Geometry check sheet. Reference: the model listing, model coordinates, mm. Coordinates: 2 decimals unless noted, no trailing zeros. Loops run counter-clockwise (first coordinate to the right, second up) from the corner with the lowest first, then second, coordinate; pieces in that order, holes last.
from build123d import *

# Parameters (mm, degrees)
F1_DEPTH  = 5.08
F2_DEPTH  = 5.08
F3_W      = 124.8834840953
F3_H      = 134.0803280473
F4_DEPTH  = 25.4
F5_DEPTH  = 1.27
F6_DEPTH  = 1.27
F8_DEPTH  = 25.4
F9_DEPTH  = 2.54
F10_DEPTH = 2.54
F11_SIZE2 = 3.418656578
F11_SIZE  = 5.6896
F12_SIZE2 = 3.6576
F12_SIZE  = 5.6322100916


with BuildPart() as f1:
    # F0 (on Front) → F1 (new body)
    with BuildSketch(Plane.XZ):
        with BuildLine():
            add(Edge.make_bspline(
                [(11.6870266183, 8.3659507286), (11.9476031572, 8.1243832132), (12.5616108346, 7.4348870399), (13.3502602627, 5.9055860485), (12.8304196463, 2.6136928469), (12.1032885822, -3.9726756525), (11.7671016032, -8.6546761386), (11.3077259518, -11.7183290107), (11.0820746049, -13.2232354954)],
                knots=[0.7644347581, 0.7644347581, 0.7644347581, 0.7644347581, 0.7813803339, 0.8102561854, 0.8494051355, 0.9057589485, 0.9537075591, 1, 1, 1, 1], degree=3))
            Line((11.6870266183, 8.3659507286), (10.7098612934, -7.1798651479))
            Line((10.7098612934, -7.1798651479), (-10.6029463932, 18.994666636))
            Line((-10.6029463932, 18.994666636), (-7.8187826003, 81.9431145827))
            add(Edge.make_bspline(
                [(-10.6029463932, 84.9773436785), (-9.8645957866, 84.411917966), (-8.8470388386, 83.6326772405), (-8.0272766718, 82.3316307612), (-7.8187826003, 81.9431145827)],
                knots=[0, 0, 0, 0, 0.0369842854, 0.0509698458, 0.0509698458, 0.0509698458, 0.0509698458], degree=3))
            add(Edge.make_bspline(
                [(-11.1952358857, -13.2855195552), (-11.1963398761, -12.8902117283), (-11.1997561984, -11.6669231231), (-11.1512885463, -5.3731858959), (-11.3422819981, 1.4393792063), (-12.1461643066, 4.6189611976), (-13.2850553088, 9.1238655935), (-15.2318124981, 13.6348809881), (-16.5294824008, 17.2010053959), (-19.3261405399, 23.6368379744), (-19.7379489625, 26.452730971), (-18.8574929103, 31.5305578619), (-16.6797816611, 35.2468825016), (-14.5909185063, 40.6408371255), (-13.4119591393, 46.1621954132), (-12.5394588361, 53.3896491248), (-12.0546254183, 59.9791874234), (-12.4642284532, 65.9827168693), (-12.3457592591, 73.9226808987), (-11.3164428193, 80.5227149139), (-11.5649092387, 84.7450814286), (-10.8268692537, 84.9232783602), (-10.6029463932, 84.9773436785)],
                knots=[0, 0, 0, 0, 0.0273896804, 0.0847579572, 0.1451631407, 0.1862204743, 0.2349457062, 0.2850522094, 0.3309978555, 0.390291, 0.4296935499, 0.4796750401, 0.527816225, 0.5818528524, 0.6365092781, 0.6980539867, 0.7565756752, 0.8124783975, 0.8767822708, 0.9378286387, 0.9811370802, 1, 1, 1, 1], degree=3))
            Line((-11.1952358857, -13.2855195552), (10.8409429303, -13.2855195552))
            add(Edge.make_bspline(
                [(10.8409429303, -13.2855195552), (10.9216527758, -13.2575733481), (11.0020770139, -13.2366740148), (11.0820746049, -13.2232354954)],
                knots=[0.9988692567, 0.9988692567, 0.9988692567, 0.9988692567, 1, 1, 1, 1], degree=3))
        make_face()
        with BuildLine():
            Line((10.7098612934, -7.1798651479), (11.6870266183, 8.3659507286))
            add(Edge.make_bspline(
                [(-7.8187826003, 81.9431145827), (-7.3326835412, 81.037298185), (-6.246332701, 78.0877738667), (-5.7619281696, 71.7972152113), (-5.7903461619, 61.0472196354), (-5.6098025476, 47.5528084715), (-5.6232359348, 35.7951775922), (-6.6035814728, 31.5572406566), (-6.642373723, 26.8588973108), (-4.7217209893, 21.7576733197), (-2.3324429206, 17.8568763905), (-0.0644904347, 14.9988475653), (2.1698029367, 12.9502128359), (5.7523840475, 11.2499433455), (8.6363164493, 10.2542124123), (10.6765655712, 9.2073747067), (11.4911211984, 8.5475648745), (11.6870266183, 8.3659507286)],
                knots=[0.0509698458, 0.0509698458, 0.0509698458, 0.0509698458, 0.0835768534, 0.1402547932, 0.2115954168, 0.293701069, 0.3674969806, 0.4121442254, 0.4580916534, 0.50894046, 0.5557476766, 0.5967458601, 0.6345135251, 0.6775157549, 0.7161326985, 0.7516948155, 0.7644347581, 0.7644347581, 0.7644347581, 0.7644347581], degree=3))
            Line((-7.8187826003, 81.9431145827), (-10.6029463932, 18.994666636))
            Line((-10.6029463932, 18.994666636), (10.7098612934, -7.1798651479))
        make_face()
        with BuildLine():
            Line((11.0820746049, -15.9663576633), (11.0820746049, -13.2855195552))
            Line((11.0820746049, -13.2855195552), (10.8409429303, -13.2855195552))
            add(Edge.make_bspline(
                [(8.3953980002, -15.9663576633), (9.1364610409, -14.6227373643), (10.004055933, -13.5752960653), (10.8409429303, -13.2855195552)],
                knots=[0.9871444865, 0.9871444865, 0.9871444865, 0.9871444865, 0.9988692567, 0.9988692567, 0.9988692567, 0.9988692567], degree=3))
            Line((8.3953980003, -15.9663576633), (11.0820746049, -15.9663576633))
        make_face()
        with BuildLine():
            add(Edge.make_bspline(
                [(8.3953980002, -15.9663576633), (9.1364610409, -14.6227373643), (10.004055933, -13.5752960653), (10.8409429303, -13.2855195552)],
                knots=[0.9871444865, 0.9871444865, 0.9871444865, 0.9871444865, 0.9988692567, 0.9988692567, 0.9988692567, 0.9988692567], degree=3))
            Line((10.8409429303, -13.2855195552), (-11.1952358857, -13.2855195552))
            Line((-11.1952358857, -13.2855195552), (-11.0308257863, -15.9663576633))
            Line((-11.0308257863, -15.9663576633), (8.3953980003, -15.9663576633))
        make_face()
        with BuildLine():
            Line((11.0820746049, -13.2855195552), (11.0820746049, -13.2232354954))
            add(Edge.make_bspline(
                [(10.8409429303, -13.2855195552), (10.9216527758, -13.2575733481), (11.0020770139, -13.2366740148), (11.0820746049, -13.2232354954)],
                knots=[0.9988692567, 0.9988692567, 0.9988692567, 0.9988692567, 1, 1, 1, 1], degree=3))
            Line((10.8409429303, -13.2855195552), (11.0820746049, -13.2855195552))
        make_face()
    extrude(amount=F1_DEPTH)

    # F2 (add): a face of the model
    f2_faces = [f1.faces().sort_by_distance(p)[0] for p in [
        (-5.0809274024, 0, 19.1888153538),
    ]]
    extrude(f2_faces, amount=F2_DEPTH)

    # F3 (on face) → F4 (cut)
    with BuildSketch(Plane.XZ.offset(5.08)):
        with Locations((7.2313416749, 30.1963053644)):
            Rectangle(F3_W, F3_H)
        with BuildLine():
            Line((-11.0308257863, -15.9663576633), (-11.1952358857, -13.2855195552))
            add(Edge.make_bspline(
                [(-11.1952358857, -13.2855195552), (-11.1963398761, -12.8902117283), (-11.1997561984, -11.6669231231), (-11.1512885463, -5.3731858959), (-11.3422819981, 1.4393792063), (-12.1461643066, 4.6189611976), (-13.2850553088, 9.1238655935), (-15.2318124981, 13.6348809881), (-16.5294824008, 17.2010053959), (-19.3261405399, 23.6368379744), (-19.7379489625, 26.452730971), (-18.8574929103, 31.5305578619), (-16.6797816611, 35.2468825016), (-14.5909185063, 40.6408371255), (-13.4119591393, 46.1621954132), (-12.5394588361, 53.3896491248), (-12.0546254183, 59.9791874234), (-12.4642284532, 65.9827168693), (-12.3457592591, 73.9226808987), (-11.3164428193, 80.5227149139), (-11.5649092387, 84.7450814286), (-10.8268692537, 84.9232783602), (-10.6029463932, 84.9773436785)],
                knots=[0, 0, 0, 0, 0.0273896804, 0.0847579572, 0.1451631407, 0.1862204743, 0.2349457062, 0.2850522094, 0.3309978555, 0.390291, 0.4296935499, 0.4796750401, 0.527816225, 0.5818528524, 0.6365092781, 0.6980539867, 0.7565756752, 0.8124783975, 0.8767822708, 0.9378286387, 0.9811370802, 1, 1, 1, 1], degree=3))
            add(Edge.make_bspline(
                [(11.0820746049, -13.2232354954), (11.3077259518, -11.7183290107), (11.7671016032, -8.6546761386), (12.1032885822, -3.9726756525), (12.8304196463, 2.6136928469), (13.3502602627, 5.9055860485), (12.443365527, 7.6641811468), (11.0743289472, 9.0032850711), (8.6363164493, 10.2542124123), (5.7523840475, 11.2499433455), (2.1698029367, 12.9502128359), (-0.0644904347, 14.9988475653), (-2.3324429206, 17.8568763905), (-4.7217209893, 21.7576733197), (-6.642373723, 26.8588973108), (-6.6035814728, 31.5572406566), (-5.6232359348, 35.7951775922), (-5.6098025476, 47.5528084715), (-5.7903461619, 61.0472196354), (-5.7619281696, 71.7972152113), (-6.2885094778, 78.6354885776), (-8.1960757736, 83.1341725308), (-9.8645957866, 84.411917966), (-10.6029463932, 84.9773436785)],
                knots=[0.7644347581, 0.7644347581, 0.7644347581, 0.7644347581, 0.810727199, 0.8586758096, 0.9150296226, 0.9541785727, 0.9830544242, 1.0127399426, 1.0483020596, 1.0869190032, 1.1299212329, 1.167688898, 1.2086870814, 1.2554942981, 1.3063431047, 1.3522905327, 1.3969377775, 1.470733689, 1.5528393413, 1.6241799649, 1.6808579047, 1.7274504726, 1.7644347581, 1.7644347581, 1.7644347581, 1.7644347581], degree=3))
            Line((11.0820746049, -13.2232354954), (11.0820746049, -15.9663576633))
            Line((11.0820746049, -15.9663576633), (-11.0308257863, -15.9663576633))
        make_face(mode=Mode.SUBTRACT)
        with BuildLine():
            add(Edge.make_bspline(
                [(-11.1952358857, -13.2855195552), (-11.1963398761, -12.8902117283), (-11.1997561984, -11.6669231231), (-11.1512885463, -5.3731858959), (-11.3422819981, 1.4393792063), (-12.1461643066, 4.6189611976), (-13.2850553088, 9.1238655935), (-15.2318124981, 13.6348809881), (-16.5294824008, 17.2010053959), (-19.3261405399, 23.6368379744), (-19.7379489625, 26.452730971), (-18.8574929103, 31.5305578619), (-16.6797816611, 35.2468825016), (-14.5909185063, 40.6408371255), (-13.4119591393, 46.1621954132), (-12.5394588361, 53.3896491248), (-12.0546254183, 59.9791874234), (-12.4642284532, 65.9827168693), (-12.3457592591, 73.9226808987), (-11.3164428193, 80.5227149139), (-11.5649092387, 84.7450814286), (-10.8268692537, 84.9232783602), (-10.6029463932, 84.9773436785)],
                knots=[0, 0, 0, 0, 0.0273896804, 0.0847579572, 0.1451631407, 0.1862204743, 0.2349457062, 0.2850522094, 0.3309978555, 0.390291, 0.4296935499, 0.4796750401, 0.527816225, 0.5818528524, 0.6365092781, 0.6980539867, 0.7565756752, 0.8124783975, 0.8767822708, 0.9378286387, 0.9811370802, 1, 1, 1, 1], degree=3))
            Line((-11.1952358857, -13.2855195552), (-11.0308257863, -15.9663576633))
            Line((-11.0308257863, -15.9663576633), (11.0820746049, -15.9663576633))
            Line((11.0820746049, -15.9663576633), (11.0820746049, -13.2232354954))
            add(Edge.make_bspline(
                [(11.0820746049, -13.2232354954), (11.3077259518, -11.7183290107), (11.7671016032, -8.6546761386), (12.1032885822, -3.9726756525), (12.8304196463, 2.6136928469), (13.3502602627, 5.9055860485), (12.443365527, 7.6641811468), (11.0743289472, 9.0032850711), (8.6363164493, 10.2542124123), (5.7523840475, 11.2499433455), (2.1698029367, 12.9502128359), (-0.0644904347, 14.9988475653), (-2.3324429206, 17.8568763905), (-4.7217209893, 21.7576733197), (-6.642373723, 26.8588973108), (-6.6035814728, 31.5572406566), (-5.6232359348, 35.7951775922), (-5.6098025476, 47.5528084715), (-5.7903461619, 61.0472196354), (-5.7619281696, 71.7972152113), (-6.2885094778, 78.6354885776), (-8.1960757736, 83.1341725308), (-9.8645957866, 84.411917966), (-10.6029463932, 84.9773436785)],
                knots=[0.7644347581, 0.7644347581, 0.7644347581, 0.7644347581, 0.810727199, 0.8586758096, 0.9150296226, 0.9541785727, 0.9830544242, 1.0127399426, 1.0483020596, 1.0869190032, 1.1299212329, 1.167688898, 1.2086870814, 1.2554942981, 1.3063431047, 1.3522905327, 1.3969377775, 1.470733689, 1.5528393413, 1.6241799649, 1.6808579047, 1.7274504726, 1.7644347581, 1.7644347581, 1.7644347581, 1.7644347581], degree=3))
        make_face()
        Polygon((-7.6687936671, 0), (0, 12.9914516583), (7.6687936671, 0), (0, -13.0022913218), align=None, mode=Mode.SUBTRACT)
    extrude(amount=-F4_DEPTH, mode=Mode.SUBTRACT)

    # F5 (add): a face of the model
    f5_faces = [f1.faces().sort_by_distance(p)[0] for p in [
        (0, -5.08, -0.0036132211),
    ]]
    extrude(f5_faces, amount=F5_DEPTH)

    # F6 (add): a face of the model
    f6_faces = [f1.faces().sort_by_distance(p)[0] for p in [
        (0, 5.08, -0.0036132211),
    ]]
    extrude(f6_faces, amount=F6_DEPTH)

    # F7 (on face) → F8 (cut)
    with BuildSketch(Plane.XZ.offset(6.35)):
        Polygon((0, -13.0022913218), (7.6687936671, 0), (0, 12.9914516583), (-7.6687936671, 0), align=None)
        Polygon((-6.6512613557, 0), (0, 10.9297530726), (6.6512613557, 0), (0, -11.3473664969), align=None, mode=Mode.SUBTRACT)
    extrude(amount=-F8_DEPTH, mode=Mode.SUBTRACT)

    # F9 (add): a face of the model
    f9_faces = [f1.faces().sort_by_distance(p)[0] for p in [
        (0, -6.35, -0.1392044748),
    ]]
    extrude(f9_faces, amount=F9_DEPTH)

    # F10 (add): a face of the model
    f10_faces = [f1.faces().sort_by_distance(p)[0] for p in [
        (0, 6.35, -0.1392044748),
    ]]
    extrude(f10_faces, amount=F10_DEPTH)

    # F11
    f11_edges = [f1.edges().sort_by_distance(p)[0] for p in [
        (3.325631, -8.89, 5.464877),
        (-3.325631, -8.89, 5.464877),
        (-3.325631, -8.89, -5.673683),
        (3.325631, -8.89, -5.673683),
    ]]
    f11_side = f1.faces().sort_by_distance((0, -8.89, -0.139204))[0]
    chamfer(f11_edges, length=F11_SIZE, length2=F11_SIZE2, reference=f11_side)

    # F12
    f12_edges = [f1.edges().sort_by_distance(p)[0] for p in [
        (3.325631, 8.89, -5.673683),
        (3.325631, 8.89, 5.464877),
        (-3.325631, 8.89, 5.464877),
        (-3.325631, 8.89, -5.673683),
    ]]
    f12_side = f1.faces().sort_by_distance((0, 8.89, -0.139204))[0]
    chamfer(f12_edges, length=F12_SIZE, length2=F12_SIZE2, reference=f12_side)


solid = f1.part
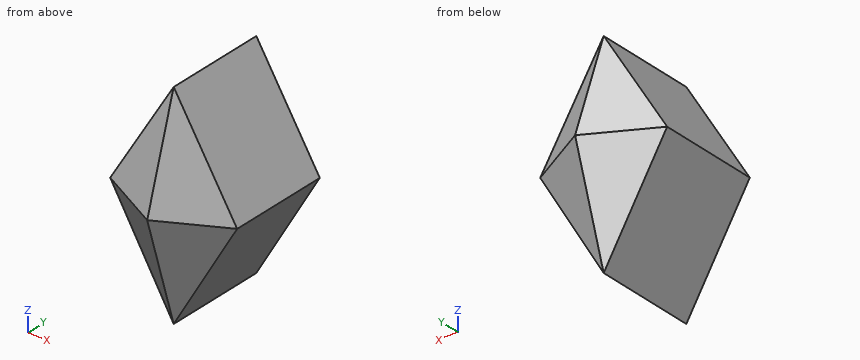
1) Section check B-B on z = -2. Record the cut outline in (x, y), and give its area (3 significant figures).
Data:
outline: (-5.48, -5.47) - (0, -8.31) - (5.48, -5.47) - (5.48, 5.23) - (0, 8.3) - (-5.48, 5.23) - close
area: 150 mm2
2) Material ranges on probe 1 along Y at (x, z) = (-0.25, 7.5); probe 2 along Z at (x, y) = (5.5, 3.25); probe 3 along X at (y, z) = (-3, -5.25), recorded low to high.
Data:
probe 1: y = -6.41 to 6.25
probe 2: z = -1.96 to 1.89
probe 3: x = -3.57 to 3.57
3) Section check A-A on x = -4.25. Record the cut outline in (y, z).
Data:
outline: (-6.71, -0.02) - (-5.47, -4.1) - (5.23, -4.1) - (6.57, -0.02) - (5.23, 3.95) - (-5.47, 3.95) - close
4) Depth check by flat-ended pin: pin 1 (6 mm diameter, centred on y = 1, z = 5, fed in from -X); pin 2 (3 mm diameter, centred on x = 4, z = -6.5, fed in from +Y); pin 3 (1 mm diameter, centred on y = -5, z = -8.5, fed in from +X). Enter the tip coordinate at first touch or a pass-through.
Data:
pin 1: stops at x = -5.43
pin 2: stops at y = 5.56
pin 3: stops at x = 1.96
5) Section check D-D on y = 7.5. Record the cut outline in (x, z), and give its area (3 significant figures).
Data:
outline: (-2.58, -0.03) - (0, -4.44) - (2.58, -0.03) - (0, 4.21) - close
area: 22.4 mm2
6) Section check C-C on y = 3. Record the cut outline in (x, z), and give its area (3 significant figures).
Data:
outline: (-6.65, 0) - (0, -11.35) - (6.65, 0) - (0, 10.93) - close
area: 148 mm2
